Read the model definition and answer for the solid it produces. Units are mm, in the model's axes. A direction names the side the tool comes from. Give positions to 0.01 mm unless a question says otherwise; leave off trailing zeros. Order: outer loops, then holes, each group sorted by start corner. A loop starts at its lowest first (then second) coordinate and runs counter-clockwise, first axis right, second up. Notation, with made-up numbers: M 13.25,-21 L 30.25,-21 A6 ccw 30.25,-14 Z; hole C -23.75,-37.75 d2. An arc over 180 degrees is marked long. One line per item, written item: value. Start each with the question number.
from build123d import *

# Parameters (mm, degrees)
SALIENTE_EXTRUIR2_DEPTH      = 1.25
SALIENTE_EXTRUIR2_DEPTH_BACK = 1.25


with BuildPart() as part:
    # Croquis1 → Saliente-Extruir2 (new, two sides: drawn at the far end of the back side and taken through both)
    with BuildSketch(Plane(origin=(0, 0, 0), x_dir=(1, 0, 0), z_dir=(0, 1, 0)).offset(-SALIENTE_EXTRUIR2_DEPTH_BACK)):
        with BuildLine():
            Line((2, 0), (14, 0))
            ThreePointArc((14, 0), (15.414213562, 0.585786438), (16, 2))
            Line((16, 2), (16, 6))
            ThreePointArc((16, 6), (15.414213562, 7.414213562), (14, 8))
            Line((14, 8), (2, 8))
            ThreePointArc((2, 8), (0.585786438, 7.414213562), (0, 6))
            Line((0, 6), (0, 2))
            ThreePointArc((0, 2), (0.585786438, 0.585786438), (2, 0))
        make_face()
        with BuildLine():
            Line((1.75, 5.75), (1.75, 2.25))
            ThreePointArc((1.75, 2.25), (1.896446609, 1.896446609), (2.25, 1.75))
            Line((2.25, 1.75), (13.75, 1.75))
            ThreePointArc((13.75, 1.75), (14.103553391, 1.896446609), (14.25, 2.25))
            Line((14.25, 2.25), (14.25, 5.75))
            ThreePointArc((14.25, 5.75), (14.103553391, 6.103553391), (13.75, 6.25))
            Line((13.75, 6.25), (2.25, 6.25))
            ThreePointArc((2.25, 6.25), (1.896446609, 6.103553391), (1.75, 5.75))
        make_face(mode=Mode.SUBTRACT)
    extrude(amount=SALIENTE_EXTRUIR2_DEPTH + SALIENTE_EXTRUIR2_DEPTH_BACK)


solid = part.part
Q1. Find section D-D, the plane x = 15.25. Give the vertices of the cut face in (y, z).
Q2. Determine the mould class of faces 3 (the flat face through (0, 0, -4)), 4 (the flat face through (8, 0, -8)), 5 (the flat face through (1.75, 0, -4)) for opening direction Z: released by +Z, released by -Z, zero draft, split by the parting line, or undercut.
Q3. Find section A-A, the plane x = 6.25. Give the vertices of the cut face in (y, z), then the cut area to 3 significant figures.
Q4. A tool of negligible diameter and unlimited length cuts with its end or side. For faces 1 (the cylindrical face through (15.43, -0.02, -7.4)), 2 (the flat face through (8, 0, -6.25)), from which of +Z, -Z, +X, -X, +Y, -Y can it reach the whole face along a straight path? Write none if from no direction.
Q5. Find section B-B, the plane y = -0.6. Give the vertices of the cut face in (x, z), then the cut area to 3 significant figures.
Q6. Find section C-C, the plane z = -2.5. Give the vertices of the cut face in (x, y).
Q7. Consider probe 1 along X at (y, z) = (-0.4, -2.5); probe 2 along Z at (x, y) = (11, 0.25). Determine where each line is inside the solid, lowest interval first.
Evaluation:
1. outline: M -1.25,-7.56 L 1.25,-7.56 L 1.25,-0.44 L -1.25,-0.44 Z
2. face 3: zero draft
2. face 4: released by -Z
2. face 5: undercut
3. outline: M -1.25,-8 L 1.25,-8 L 1.25,-6.25 L -1.25,-6.25 Z; M -1.25,-1.75 L 1.25,-1.75 L 1.25,0 L -1.25,0 Z
3. area: 8.75 mm2
4. face 1: -Z, +X, +Y, -Y
4. face 2: +Y, -Y
5. outline: M 0,-6 A2 ccw 2,-8 L 14,-8 A2 ccw 16,-6 L 16,-2 A2 ccw 14,0 L 2,0 A2 ccw 0,-2 Z; hole M 1.75,-5.75 A0.5 ccw 2.25,-6.25 L 13.75,-6.25 A0.5 ccw 14.25,-5.75 L 14.25,-2.25 A0.5 ccw 13.75,-1.75 L 2.25,-1.75 A0.5 ccw 1.75,-2.25 Z
5. area: 68.5 mm2
6. outline: M 0,-1.25 L 1.75,-1.25 L 1.75,1.25 L 0,1.25 Z; M 14.25,-1.25 L 16,-1.25 L 16,1.25 L 14.25,1.25 Z
7. probe 1: 0 to 1.75, 14.25 to 16
7. probe 2: -8 to -6.25, -1.75 to 0
